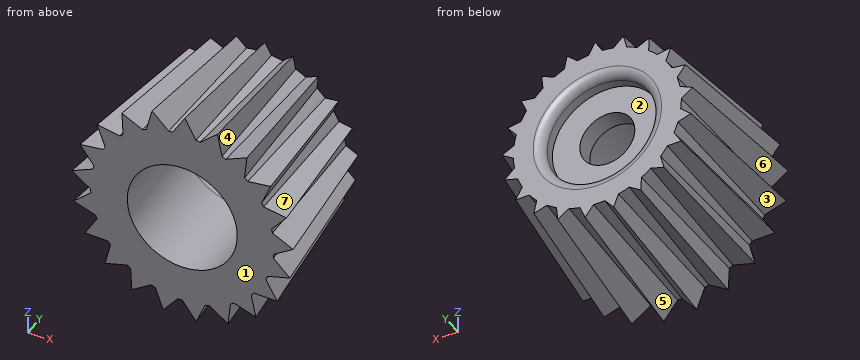
```python
from build123d import *

# Parameters (mm, degrees)
BOSS_EXTRUDE1_DEPTH = 8
BOSS_EXTRUDE1_DRAFT = 3
SKETCH2_R           = 3
CUT_EXTRUDE1_DEPTH  = 6
SKETCH3_R           = 1.5
CUT_EXTRUDE2_DEPTH  = 6
FILLET3_R           = 0.5
CUT_EXTRUDE3_START  = -1
SKETCH4_R           = 3
CUT_EXTRUDE3_DEPTH  = 1
FILLET4_R           = 0.5


with BuildPart() as part:
    # Sketch1 → Boss-Extrude1 (with draft: the straight prism first)
    with BuildSketch(Plane(origin=(0, 0, 0), x_dir=(1, 0, 0), z_dir=(0, 1, 0))):
        with BuildLine():
            ThreePointArc((0, 5), (-0.115399429, 4.99866812), (-0.230737379, 4.994673189))
            Line((-0.230737379, 4.994673189), (-1.040018866, 5.962771522))
            Line((-1.040018866, 5.962771522), (-1.473775872, 4.777864029))
            ThreePointArc((-1.473775872, 4.777864029), (-1.58365585, 4.742576742), (-1.692692132, 4.704762837))
            Line((-1.692692132, 4.704762837), (-2.751371505, 5.391311371))
            Line((-2.751371505, 5.391311371), (-2.81660029, 4.131193872))
            ThreePointArc((-2.81660029, 4.131193872), (-2.911197498, 4.065086607), (-3.00424376, 3.99681366))
            Line((-3.00424376, 3.99681366), (-4.218252713, 4.340809546))
            Line((-4.218252713, 4.340809546), (-3.909157412, 3.117449009))
            ThreePointArc((-3.909157412, 3.117449009), (-3.980066474, 3.026395689), (-4.048855146, 2.93373005))
            Line((-4.048855146, 2.93373005), (-5.310323655, 2.904607743))
            Line((-5.310323655, 2.904607743), (-4.654368743, 1.826705122))
            ThreePointArc((-4.654368743, 1.826705122), (-4.695289077, 1.718796232), (-4.733707985, 1.60997165))
            Line((-4.733707985, 1.60997165), (-5.930549036, 1.210318796))
            Line((-5.930549036, 1.210318796), (-4.986018986, 0.373650468))
            ThreePointArc((-4.986018986, 0.373650468), (-4.99331464, 0.258474187), (-4.997950095, 0.143160204))
            Line((-4.997950095, 0.143160204), (-6.02381911, -0.591512288))
            Line((-6.02381911, -0.591512288), (-4.874639561, -1.11260467))
            ThreePointArc((-4.874639561, -1.11260467), (-4.847662285, -1.224814423), (-4.818102407, -1.336371654))
            Line((-4.818102407, -1.336371654), (-5.581846421, -2.340784909))
            Line((-5.581846421, -2.340784909), (-4.330127019, -2.5))
            ThreePointArc((-4.330127019, -2.5), (-4.271273862, -2.599272897), (-4.210145176, -2.697161026))
            Line((-4.210145176, -2.697161026), (-4.643902182, -3.882068519))
            Line((-4.643902182, -3.882068519), (-3.400863689, -3.665259359))
            ThreePointArc((-3.400863689, -3.665259359), (-3.315364013, -3.742774568), (-3.228098069, -3.818295805))
            Line((-3.228098069, -3.818295805), (-3.293326854, -5.078413304))
            Line((-3.293326854, -5.078413304), (-2.169418696, -4.50484434))
            ThreePointArc((-2.169418696, -4.50484434), (-2.064869521, -4.553714293), (-1.959220284, -4.600158245))
            Line((-1.959220284, -4.600158245), (-1.650124983, -5.823518782))
            Line((-1.650124983, -5.823518782), (-0.745211331, -4.944154131))
            ThreePointArc((-0.745211331, -4.944154131), (-0.630902312, -4.960036519), (-0.516257178, -4.973276438))
            Line((-0.516257178, -4.973276438), (0.139697734, -6.051179059))
            Line((0.139697734, -6.051179059), (0.745211331, -4.944154131))
            ThreePointArc((0.745211331, -4.944154131), (0.859123337, -4.925637734), (0.972577644, -4.904497194))
            Line((0.972577644, -4.904497194), (1.917107695, -5.741165522))
            Line((1.917107695, -5.741165522), (2.169418696, -4.50484434))
            ThreePointArc((2.169418696, -4.50484434), (2.272812107, -4.453574421), (2.374994674, -4.399931852))
            Line((2.374994674, -4.399931852), (3.524174223, -4.921024233))
            Line((3.524174223, -4.921024233), (3.400863689, -3.665259359))
            ThreePointArc((3.400863689, -3.665259359), (3.484551548, -3.585791476), (3.566383005, -3.504413255))
            Line((3.566383005, -3.504413255), (4.818102407, -3.663628346))
            Line((4.818102407, -3.663628346), (4.330127019, -2.5))
            ThreePointArc((4.330127019, -2.5), (4.386673291, -2.399395223), (4.440882555, -2.297512163))
            Line((4.440882555, -2.297512163), (5.683921048, -2.080703003))
            Line((5.683921048, -2.080703003), (4.874639561, -1.11260467))
            ThreePointArc((4.874639561, -1.11260467), (4.899019862, -0.999802174), (4.920790201, -0.886467032))
            Line((4.920790201, -0.886467032), (6.04469836, -0.312898067))
            Line((6.04469836, -0.312898067), (4.986018986, 0.373650468))
            ThreePointArc((4.986018986, 0.373650468), (4.97606702, 0.488627685), (4.963464044, 0.603344585))
            Line((4.963464044, 0.603344585), (5.868377696, 1.482709236))
            Line((5.868377696, 1.482709236), (4.654368743, 1.826705122))
            ThreePointArc((4.654368743, 1.826705122), (4.610968785, 1.933640831), (4.565112324, 2.039546388))
            Line((4.565112324, 2.039546388), (5.170625921, 3.146571316))
            Line((5.170625921, 3.146571316), (3.909157412, 3.117449009))
            ThreePointArc((3.909157412, 3.117449009), (3.836165739, 3.206841502), (3.761130341, 3.294525544))
            Line((3.761130341, 3.294525544), (4.013441342, 4.530846726))
            Line((4.013441342, 4.530846726), (2.81660029, 4.131193872))
            ThreePointArc((2.81660029, 4.131193872), (2.720502533, 4.195100234), (2.622955421, 4.256771647))
            Line((2.622955421, 4.256771647), (2.499644887, 5.512536521))
            Line((2.499644887, 5.512536521), (1.473775872, 4.777864029))
            ThreePointArc((1.473775872, 4.777864029), (1.363110737, 4.810605899), (1.251719402, 4.840784909))
            Line((1.251719402, 4.840784909), (0.763744014, 6.004413255))
            Line((0.763744014, 6.004413255), (0, 5))
        make_face()
    extrude(amount=BOSS_EXTRUDE1_DEPTH)
    # Boss-Extrude1: the draft: its side faces are tilted about the plane it starts from
    boss_extrude1_sides = [part.faces().sort_by_distance(p)[0] for p in [
        (4.867869122, 4, -2.593058852),
        (4.539891667, 4, -3.132010163),
        (3.836165739, 4, -3.206841502),
        (3.887285841, 4, -3.912686135),
        (3.415020816, 4, -4.331020299),
        (2.720502533, 4, -4.195100234),
        (2.561300154, 4, -4.884654084),
        (1.98671038, 4, -5.145200275),
        (1.363110737, 4, -4.810605899),
        (1.007731708, 4, -5.422599082),
        (0.381872007, 4, -5.502206628),
        (-0.115399429, 4, -4.99866812),
        (-0.635378122, 4, -5.478722355),
        (-1.256897369, 4, -5.370317775),
        (-1.58365585, 4, -4.742576742),
        (-2.222031818, 4, -5.048037104),
        (-2.783985898, 4, -4.761252621),
        (-2.911197498, 4, -4.065086607),
        (-3.611248236, 4, -4.168811603),
        (-4.063705062, 4, -3.729129278),
        (-3.980066474, 4, -3.026395689),
        (-4.679589401, 4, -2.919168896),
        (-4.982346199, 4, -2.365656432),
        (-4.695289077, 4, -1.718796232),
        (-5.332128511, 4, -1.410145223),
        (-5.458284011, 4, -0.791984632),
        (-4.99331464, 4, -0.258474187),
        (-5.510884603, 4, 0.224176042),
        (-5.449229336, 4, 0.852058479),
        (-4.847662285, 4, 1.224814423),
        (-5.199974414, 4, 1.838578282),
        (-4.95598672, 4, 2.420392455),
        (-4.271273862, 4, 2.599272897),
        (-4.427023679, 4, 3.289614773),
        (-4.022382935, 4, 3.773663939),
        (-3.315364013, 4, 3.742774568),
        (-3.260712462, 4, 4.448354555),
        (-2.731372775, 4, 4.791628822),
        (-2.064869521, 4, 4.553714293),
        (-1.804672633, 4, 5.211838513),
        (-1.197668157, 4, 5.383836456),
        (-0.630902312, 4, 4.960036519),
        (-0.188279722, 4, 5.512227748),
        (0.442454532, 4, 5.497666595),
        (0.859123337, 4, 4.925637734),
        (1.444842669, 4, 5.322831358),
        (2.043263195, 4, 5.123004931),
        (2.272812107, 4, 4.453574421),
        (2.949584449, 4, 4.660478042),
        (3.462518956, 4, 4.293141796),
        (3.484551548, 4, 3.585791476),
        (4.192242706, 4, 3.584020801),
        (4.574114713, 4, 3.081814173),
        (4.386673291, 4, 2.399395223),
        (5.062401801, 4, 2.189107583),
        (5.279280304, 4, 1.596653836),
        (4.899019862, 4, 0.999802174),
        (5.48274428, 4, 0.599682549),
        (5.515358673, 4, -0.030376201),
        (4.97606702, 4, -0.488627685),
        (5.41592087, 4, -1.043026911),
        (5.26137322, 4, -1.654707179),
        (4.610968785, 4, -1.933640831),
    ]]
    draft(boss_extrude1_sides, Plane(origin=(0, 0, 0), x_dir=(1, 0, 0), z_dir=(0, 1, 0)), BOSS_EXTRUDE1_DRAFT)

    # Sketch2 → Cut-Extrude1 (cut)
    with BuildSketch(Plane.XZ):
        with Locations(Location((0, 0, 0), (0, 0, 270))):
            Circle(SKETCH2_R)
    extrude(amount=-CUT_EXTRUDE1_DEPTH, mode=Mode.SUBTRACT)

    # Sketch3 → Cut-Extrude2 (cut)
    with BuildSketch(Plane.XZ.offset(-6)):
        with Locations(Location((0, 0, 0), (0, 0, 270))):
            Circle(SKETCH3_R)
    extrude(amount=-CUT_EXTRUDE2_DEPTH, mode=Mode.SUBTRACT)

    # Fillet3
    fillet3_edges = [part.edges().sort_by_distance(p)[0] for p in [
        (0, 6, 3),
    ]]
    fillet(fillet3_edges, radius=FILLET3_R)

    # Sketch4 → Cut-Extrude3 (cut)
    with BuildSketch(Plane(origin=(0, 8, 0), x_dir=(1, 0, 0), z_dir=(0, 1, 0)).offset(CUT_EXTRUDE3_START)):
        with Locations(Location((0, 0, 0), (0, 0, 90))):
            Circle(SKETCH4_R)
    extrude(amount=CUT_EXTRUDE3_DEPTH, mode=Mode.SUBTRACT)

    # Fillet4
    fillet4_edges = [part.edges().sort_by_distance(p)[0] for p in [
        (0, 8, 3),
    ]]
    fillet(fillet4_edges, radius=FILLET4_R)


solid = part.part
```
CAD build for the part. Positions are in the model's coordinates, mm. Face numbers are marked on the shaded views. A direction names the side the tool comes from. Coordinates: 2 decimals unless noted, no trailing zeros. Use one line per item in the form item = value. Start each with the question number.
1) Pull direction X, two halves, no side cores. Call the marked faces 1, 2 and 3: +X half, -X half, draft (parallel to the pull), parting line (faces both ways), or undercut.
2) Drill centre lines: L1, parallel to Z at x = -4.75, y = 3.75; L2, parallel to Y at x = -2.5, z = -0.5; L3, parallel to X at y = 7.25, z = 0. Where is each one in solid material? Low to high. Write a range as [from, to].
3) Tool access for the marked faces 4, 5, 6 and 7: list every direction of +Z, -Z, +X, -X, +Y, -Y with a clear straight run to the whole face (end or side of a thin tool).
4) Drop flat-ended pins along their axis: pin 1 (1.8 mm diameter, centred on x = -1, z = -1, fed in from +Y); pin 2 (1.5 mm diameter, centred on x = -1, z = 0, fed in from -Y). Give the stop position or say it passes through.
Entries:
q1.face_1 = draft
q1.face_2 = undercut
q1.face_3 = -X half
q2.L1 = [-2.72, -2.36], [-1.4, 0.95], [1.57, 2.25]
q2.L2 = [6, 7]
q2.L3 = [-4.62, -3], [3, 4.86]
q3.face_4 = +Z, +Y
q3.face_5 = -Z, +Y
q3.face_6 = -X, +Y
q3.face_7 = +X, +Y
q4.pin_1 = 7
q4.pin_2 = 6
